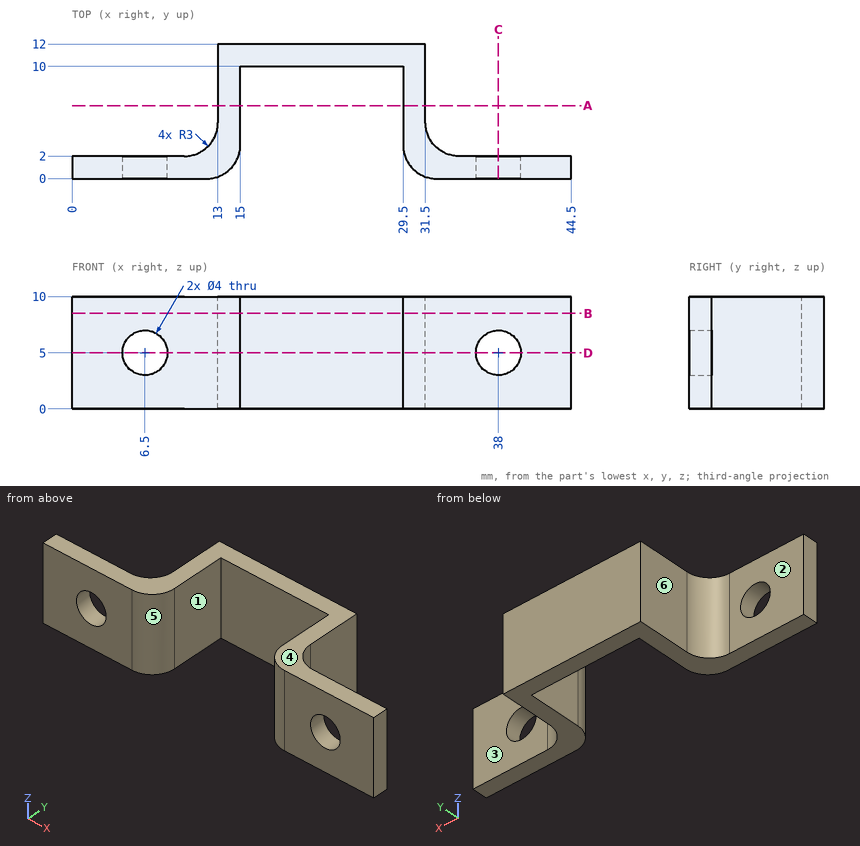
The drawing under review shows one solid part. Ordinate dimensions are in mm from its lowest x, y, z. A direction names the side the tool comes from. Coordinates: 2 decimals unless noted, no trailing zeros. Loops run counter-clockwise (first coordinate to the right, second up) from the corner with the lowest first, then second, coordinate; pieces in that order, holes last. Notation, with made-up numbers: (15, 15) -> (57, 15) arc R13 ccw to (57, 27) -> close; hole circle Ø10 at (-10.75, 82). An arc over 180 degrees is marked (long way). Answer as a JSON object with one key per item and string values.
Q1. To check wall thickness, follow L1, parallel to X at y = 5.75, z = 6.75; L2, parallel to Z at x = 6.5, y = 0.8; L3, parallel to X at y = 3, z = 9. State the ranges of each line that lie inside material, in increasing order.
Answer block:
{"L1": "x = 13 to 15, 29.5 to 31.5", "L2": "z = 0 to 3, 7 to 10", "L3": "x = 12.24 to 15, 29.5 to 32.26"}
Q2. Take a section at D-D on z = 5. Give the boundary of the cut face in (x, y).
Answer block:
{"outline": "(0, 0) -> (4.5, 0) -> (4.5, 2) -> (0, 2) -> close; (8.5, 0) -> (12, 0) arc R3 ccw to (15, 3) -> (15, 10) -> (29.5, 10) -> (29.5, 3) arc R3 ccw to (32.5, 0) -> (36, 0) -> (36, 2) -> (34.5, 2) arc R3 cw to (31.5, 5) -> (31.5, 12) -> (13, 12) -> (13, 5) arc R3 cw to (10, 2) -> (8.5, 2) -> close; (40, 0) -> (44.5, 0) -> (44.5, 2) -> (40, 2) -> close"}
Q3. Tool access review of the marked faces 1, 2 and 3: name each direction out of +Z, -Z, +X, -X, +Y, -Y from which nothing blocks a thin tool from reaching the whole face with its end or side.
Answer block:
{"face 1": "+Z, -Z, -Y", "face 2": "+Z, -Z, -X, +Y", "face 3": "+Z, -Z, +X, +Y"}
Q4. Clearance check with flat-ended pins moving along their axes: pin 1 Ø6 at (x, z) = (39, 5.5) entering from -Y; pin 2 Ø1 at (x, z) = (8, 9) entering from +Y; pin 3 Ø2 at (y, z) = (10.5, 8) entering from +X; pin 4 Ø2 at (y, z) = (7, 5) entering from -X. State where each tip first meets the part, or that it passes through.
Answer block:
{"pin 1": "stops at y = 0", "pin 2": "stops at y = 2", "pin 3": "stops at x = 31.5", "pin 4": "stops at x = 13"}
Q5. The part is to be moulded in two halves that separate along X. For the marked faces 4, 5 and 6, say which applies: +X half, -X half, draft (parallel to the pull), parting line (faces both ways), or undercut.
Answer block:
{"face 4": "draft", "face 5": "undercut", "face 6": "-X half"}
Q6. Take a section at B-B on z = 8.5. Give the boundary of the cut face in (x, y), plus the area to 3 significant figures.
Answer block:
{"outline": "(0, 0) -> (12, 0) arc R3 ccw to (15, 3) -> (15, 10) -> (29.5, 10) -> (29.5, 3) arc R3 ccw to (32.5, 0) -> (44.5, 0) -> (44.5, 2) -> (34.5, 2) arc R3 cw to (31.5, 5) -> (31.5, 12) -> (13, 12) -> (13, 5) arc R3 cw to (10, 2) -> (0, 2) -> close", "area": "129 mm^2"}
Q7. Take a section at C-C on x = 38. Give the boundary of the cut face in (y, z).
Answer block:
{"outline": "(0, 0) -> (2, 0) -> (2, 3) -> (0, 3) -> close; (0, 7) -> (2, 7) -> (2, 10) -> (0, 10) -> close"}
Q8. Take a section at A-A on y = 6.5. Give the boundary of the cut face in (x, z), plus the area to 3 significant figures.
Answer block:
{"outline": "(13, 0) -> (15, 0) -> (15, 10) -> (13, 10) -> close; (29.5, 0) -> (31.5, 0) -> (31.5, 10) -> (29.5, 10) -> close", "area": "40.0 mm^2"}
